Work out the finished part from the listing and answer in its coordinate system (mm). A direction names the side the tool comes from. Coordinates: 2 decimals unless noted, no trailing zeros. Loops run counter-clockwise (first coordinate to the right, second up) from the corner with the lowest first, then second, coordinate; pieces in that order, holes last. Notation, with made-up numbers: (-13.75, 57) - (19.25, 57) arc R22 cw to (19.25, 81) - close; hole circle Ø7 at (27.25, 77). An arc over 180 degrees is marked (long way). Write each question's results on one line, items separated by ' | '. Start each with the question number.
Item 1: For a pull along Y with two mould halves and no side action, classify faces 1 (the face through (-470, 470, -450)), 2 (the face through (470, -440, -222)), 3 (the face through (-35, 500, 5)) as +Y half, -Y half, draft (parallel to the pull), parting line (faces both ways), or undercut.
Item 2: Consider probe 1 along Z at (x, y) = (-457, 37); probe 2 along Y at (x, z) = (447.5, -268.5). Determine where each line is inside the solid, lowest interval first. Write a range as [from, to].
Item 3: Section B-B, the plane x = 374 is taken. Write down the section's boundary in (y, z).
Item 4: A tool of negligible diameter and unlimited length cuts with its end or side. For faces 4 (the face through (-470, -470, -450)), 5 (the face through (440, -470, -222)), 6 (the face through (-470, -440, -222)), from which of +Z, -Z, +X, -X, +Y, -Y can it reach the whole face along a straight path? Write none if from no direction.
Item 5: Section A-A, the plane z = -104 is taken. Write down the section's boundary in (x, y).
Item 6: This flat-tipped pin is pushed along its axis until it touches: pin 1 Ø5 at (x, y) = (-355, 233.5) entering from -Z. Where does it stop, or does it pass through?
from build123d import *

# Parameters (mm, degrees)
F0_W            = 1000
F0_H            = 1000
F1_DEPTH        = 120
F2_W            = 60
F2_H            = 60
F3_DEPTH        = 450
F3_COPIES_COUNT = 4


# Not quite as in the source:
# - a pattern or mirror of a feature is missing from the dataset's text; its kind, count and spacing are read off the source's solid


with BuildPart() as f1:
    # F0 (on Top) → F1 (new body)
    with BuildSketch(Plane.XY):
        Rectangle(F0_W, F0_H)
    extrude(amount=F1_DEPTH)

    # F2 (on face) → F3 (join)
    with BuildSketch(Plane(origin=(0, 0, 0), x_dir=(1, 0, 0), z_dir=(0, 0, -1))):
        with Locations((-470, 470)):
            Rectangle(F2_W, F2_H)
    f3 = extrude(amount=F3_DEPTH)

    # F3_copies: F3 ×4 about axis
    f3_copies_axis = Axis((0, 0, 0), (0, 0, 1))
    for i in range(1, F3_COPIES_COUNT):
        add(f3.rotate(f3_copies_axis, i * 360 / F3_COPIES_COUNT))


solid = f1.part
Answer key:
1) face 1: draft | face 2: undercut | face 3: +Y half
2) probe 1: z = [0, 120] | probe 2: y = [-500, -440], [440, 500]
3) outline: (-500, 0) - (500, 0) - (500, 120) - (-500, 120) - close
4) face 4: -Z, +X, -X, +Y, -Y | face 5: -Z, +Y, -Y | face 6: -Z, +X, -X
5) outline: (-500, -500) - (-440, -500) - (-440, -440) - (-500, -440) - close; (-500, 440) - (-440, 440) - (-440, 500) - (-500, 500) - close; (440, -500) - (500, -500) - (500, -440) - (440, -440) - close; (440, 440) - (500, 440) - (500, 500) - (440, 500) - close
6) pin 1: stops at z = 0
